Input: part model. Units: mm. Frame: model coordinates. A direction names the side the tool comes from. Give positions to 0.01 mm unless a question says otherwise; leave off trailing zeros. Loops run counter-clockwise (first coordinate to the right, second up) from the corner with the lowest first, then second, coordinate; pieces in that order, holes last.
from build123d import *

# Parameters (mm, degrees)
BOSS_EXTRUDE1_DEPTH = 4.5
SKETCH3_W           = 6.5
SKETCH3_H           = 20
SKETCH3_R           = 2.15265
BOSS_EXTRUDE2_DEPTH = 4.7625
CUT_EXTRUDE1_DEPTH  = 2.5
FILLET1_R           = 4


with BuildPart() as part:
    # Sketch1 → Boss-Extrude1 (new, symmetric)
    with BuildSketch(Plane(origin=(0, 0, 0), x_dir=(0, 0, -1), z_dir=(1, 0, 0))):
        Polygon((5.9, 2.2625), (5.9, 4.7625), (4.1, 4.7625), (4.1, 2.2625), (0.9, 2.2625), (0.9, 4.7625), (0, 4.7625), (0, 0), (20, 0), (20, 4.7625), (19.1, 4.7625), (19.1, 2.2625), (15.9, 2.2625), (15.9, 4.7625), (14.1, 4.7625), (14.1, 2.2625), (10.9, 2.2625), (10.9, 4.7625), (9.1, 4.7625), (9.1, 2.2625), align=None)
    extrude(amount=BOSS_EXTRUDE1_DEPTH, both=True)

    # Sketch3 → Boss-Extrude2 (add)
    # profile 1 of 2: a face of its own
    with BuildSketch(Plane.XZ):
        with Locations((7.75, -10)):
            Rectangle(SKETCH3_W, SKETCH3_H)
        with Locations(Location((8, -10, 0), (0, 0, 270))):
            Circle(SKETCH3_R, mode=Mode.SUBTRACT)
    # profile 2 of 2: a face of its own
    with BuildSketch(Plane.XZ):
        with Locations((-7.75, -10)):
            Rectangle(SKETCH3_W, SKETCH3_H)
        with Locations(Location((-8, -10, 0), (0, 0, 270))):
            Circle(SKETCH3_R, mode=Mode.SUBTRACT)
    extrude(amount=-BOSS_EXTRUDE2_DEPTH)

    # Sketch4 → Cut-Extrude1 (cut)
    with BuildSketch(Plane(origin=(0, 4.7625, 0), x_dir=(1, 0, 0), z_dir=(0, 1, 0))):
        with BuildLine():
            Line((4.5, 0.9), (4.5, 4.1))
            ThreePointArc((4.5, 4.1), (6.1, 2.5), (4.5, 0.9))
        make_face()
        with BuildLine():
            Line((4.5, 5.9), (4.5, 9.1))
            ThreePointArc((4.5, 9.1), (6.1, 7.5), (4.5, 5.9))
        make_face()
        with BuildLine():
            Line((4.5, 10.9), (4.5, 14.1))
            ThreePointArc((4.5, 14.1), (6.1, 12.5), (4.5, 10.9))
        make_face()
        with BuildLine():
            Line((4.5, 15.9), (4.5, 19.1))
            ThreePointArc((4.5, 19.1), (6.1, 17.5), (4.5, 15.9))
        make_face()
        with BuildLine():
            Line((-4.5, 15.9), (-4.5, 19.1))
            ThreePointArc((-4.5, 19.1), (-6.1, 17.5), (-4.5, 15.9))
        make_face()
        with BuildLine():
            Line((-4.5, 10.9), (-4.5, 14.1))
            ThreePointArc((-4.5, 14.1), (-6.1, 12.5), (-4.5, 10.9))
        make_face()
        with BuildLine():
            Line((-4.5, 5.9), (-4.5, 9.1))
            ThreePointArc((-4.5, 9.1), (-6.1, 7.5), (-4.5, 5.9))
        make_face()
        with BuildLine():
            Line((-4.5, 0.9), (-4.5, 4.1))
            ThreePointArc((-4.5, 4.1), (-6.1, 2.5), (-4.5, 0.9))
        make_face()
    extrude(amount=-CUT_EXTRUDE1_DEPTH, mode=Mode.SUBTRACT)

    # Fillet1
    fillet1_edges = [part.edges().sort_by_distance(p)[0] for p in [
        (11, 2.38125, 0),
        (11, 2.38125, -20),
        (-11, 2.38125, -20),
        (-11, 2.38125, 0),
    ]]
    fillet(fillet1_edges, radius=FILLET1_R)


solid = part.part
(1) Mould query, pull axis X, two halves, no side actions, for faces 1 (the flat face through (0, 3, -10.9)), 2 (the flat face through (0, 2, 0)), 3 (the cylindrical face through (-9.797, 2.415, -18.859)), 4 (the flat face through (0, 2.262, -3)). Classes: +X half, -X half, draft (parallel to the pull), parting line (faces both ways), or undercut.
Values follow:
face 1: undercut
face 2: draft
face 3: -X half
face 4: undercut
(2) Ray query, probe 1 along X at (y, z) = (1.2, -10); probe 2 along Z at (x, y) = (-4.5, 2.5); probe 3 along Y at (x, z) = (-4.5, -3). Return the intervals inside material, ascending.
Values follow:
probe 1: x = -11 to -10.15, -5.85 to 5.85, 10.15 to 11
probe 2: z = -20 to -19.1, -15.9 to -14.1, -10.9 to -9.1, -5.9 to -4.1, -0.9 to 0
probe 3: y = 0 to 2.26
(3) Reachability of faces 5 (the cylindrical face through (-9.859, 2.415, -1.203)), 6 (the flat face through (0, 3, -15.9)) from +Z, -Z, +X, -X, +Y, -Y: full face, straight path, thin tool, end or side. Return the list, or none.
Values follow:
face 5: +Z, -X, +Y, -Y
face 6: +Y
(4) Cut plane C-C (x = -4). Return the cut outline in (y, z), and give its area (4 significant figures).
Values follow:
outline: (0, -20) - (4.76, -20) - (4.76, -19.1) - (2.26, -19.1) - (2.26, -15.9) - (4.76, -15.9) - (4.76, -14.1) - (2.26, -14.1) - (2.26, -10.9) - (4.76, -10.9) - (4.76, -9.1) - (2.26, -9.1) - (2.26, -5.9) - (4.76, -5.9) - (4.76, -4.1) - (2.26, -4.1) - (2.26, -0.9) - (4.76, -0.9) - (4.76, 0) - (0, 0) - close
area: 63.25 mm2
(5) Cut plane A-A (z = -10). Return the cut outline in (x, y).
Values follow:
outline: (-11, 0) - (-10.15, 0) - (-10.15, 4.76) - (-11, 4.76) - close; (-5.85, 0) - (5.85, 0) - (5.85, 4.76) - (-5.85, 4.76) - close; (10.15, 0) - (11, 0) - (11, 4.76) - (10.15, 4.76) - close
(6) Pin query (flat end, axial travel): pin 1 Ø1 at (x, z) = (2.5, -12) entering from +Y. Return the tip coordinate at first contact, or that it passes through.
Values follow:
pin 1: stops at y = 2.26
(7) Cut plane B-B (y = 4). Return the cut outline in (x, z).
Values follow:
outline: (-11, -16) arc R4 ccw to (-7, -20) - (7, -20) arc R4 ccw to (11, -16) - (11, -4) arc R4 ccw to (7, 0) - (-7, 0) arc R4 ccw to (-11, -4) - close; hole circle Ø4.31 at (-8, -10); hole (-4.5, -19.1) - (4.5, -19.1) arc R1.6 ccw to (4.5, -15.9) - (-4.5, -15.9) arc R1.6 ccw to start; hole (-4.5, -14.1) - (4.5, -14.1) arc R1.6 ccw to (4.5, -10.9) - (-4.5, -10.9) arc R1.6 ccw to start; hole (-4.5, -9.1) - (4.5, -9.1) arc R1.6 ccw to (4.5, -5.9) - (-4.5, -5.9) arc R1.6 ccw to start; hole (-4.5, -4.1) - (4.5, -4.1) arc R1.6 ccw to (4.5, -0.9) - (-4.5, -0.9) arc R1.6 ccw to start; hole circle Ø4.31 at (8, -10)
(8) Cut plane D-D (y = 0.9). Return the cut outline in (x, z), and give its area (3 significant figures).
Values follow:
outline: (-11, -16) arc R4 ccw to (-7, -20) - (7, -20) arc R4 ccw to (11, -16) - (11, -4) arc R4 ccw to (7, 0) - (-7, 0) arc R4 ccw to (-11, -4) - close; hole circle Ø4.31 at (-8, -10); hole circle Ø4.31 at (8, -10)
area: 397 mm2
